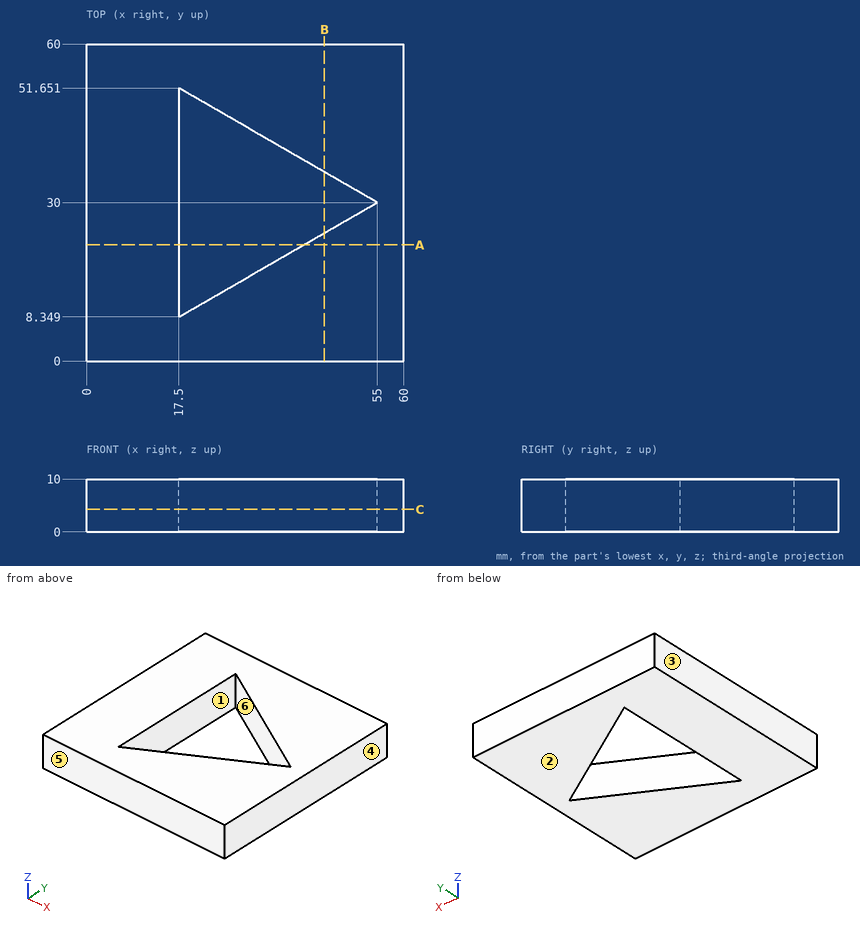
Input: dimensioned drawing with shaded views. Units: mm. Origin: part minimum x, y, z. A direction names the side the tool comes from. Coordinates: 2 decimals unless noted, no trailing zeros. Loops run counter-clockwise (first coordinate to the right, second up) from the corner with the lowest first, then second, coordinate; pieces in that order, holes last. Notation, with made-up numbers: M -15,-16 L 35,-16 A12 ccw 35,-7 Z; hole C 4,44 d7. An arc over 180 degrees is marked long. One line per item, written item: value.
(1) Section B-B (x = 45). Output: boundary loops of the cut face in (y, z).
Filled in:
outline: M 0,0 L 24.23,0 L 24.23,10 L 0,10 Z; M 35.77,0 L 60,0 L 60,10 L 35.77,10 Z
(2) Pin query (flat end, axial travel): pin 1 (8 mm diameter, centred on x = 23, y = 20.5, fed in from +Z). Return the tip coordinate at first contact, or that it passes through.
Filled in:
pin 1: through
(3) Line query: line 1 along X through (y, z) = (16, 6); line 2 along X through (y, z) = (32, 5.75) (1 decimal); line 3 along Y through (x, z) = (45, 8.5) (1 decimal). Output: solid intervals per line, ascending. Write a range as from..to.
Filled in:
line 1: 0..17.5, 30.75..60
line 2: 0..17.5, 51.5..60
line 3: 0..24.2, 35.8..60
(4) Section C-C (z = 4.25). Output: boundary loops of the cut face in (x, y), and give its area (3 significant figures).
Filled in:
outline: M 0,0 L 60,0 L 60,60 L 0,60 Z; hole M 17.5,8.35 L 55,30 L 17.5,51.65 Z
area: 2,790 mm^2
(5) Pull-direction query (X, two-part tool) for the marked faces 1, 2, 3 and 4; classes: +X half, -X half, draft (parallel to the pull), parting line (faces both ways), or undercut.
Filled in:
face 1: undercut
face 2: draft
face 3: -X half
face 4: +X half
(6) Reachability of the marked faces 5 and 6 from +Z, -Z, +X, -X, +Y, -Y: full face, straight path, thin tool, end or side. Return the list, or none.
Filled in:
face 5: +Z, -Z, +X, -X, -Y
face 6: +Z, -Z
(7) Section A-A (y = 22). Output: boundary loops of the cut face in (x, z).
Filled in:
outline: M 0,0 L 17.5,0 L 17.5,10 L 0,10 Z; M 41.14,0 L 60,0 L 60,10 L 41.14,10 Z
